from build123d import *

# Parameters (mm, degrees)
SKETCH1_R           = 1.35
BOSS_EXTRUDE1_DEPTH = 10
SKETCH2_R           = 25
BOSS_EXTRUDE2_DEPTH = 2
CIRPATTERN1_COUNT   = 2
CIRPATTERN1_ANGLE   = 134.8
CIRPATTERN2_COUNT   = 2
CIRPATTERN2_ANGLE   = 225.2
FILLET1_R           = 7


with BuildPart() as part:
    # Sketch1 → Boss-Extrude1 (new body)
    with BuildSketch(Plane.XY):
        with BuildLine():
            Line((3.15, 3.85), (3.15, -1.35))
            ThreePointArc((3.15, -1.35), (0, -4.5), (-3.15, -1.35))
            Line((-3.15, -1.35), (-3.15, 3.85))
            ThreePointArc((-3.15, 3.85), (0, 7), (3.15, 3.85))
        make_face()
        Circle(SKETCH1_R, mode=Mode.SUBTRACT)
    boss_extrude1 = extrude(amount=BOSS_EXTRUDE1_DEPTH)

    # Sketch2 → Boss-Extrude2 (add)
    with BuildSketch(Plane.XY.offset(10)):
        with Locations((0, 26.766568047)):
            Circle(SKETCH2_R)
    extrude(amount=-BOSS_EXTRUDE2_DEPTH)

    # CirPattern1: Boss-Extrude1 ×2 about axis
    cirpattern1_axis = Axis((0, 26.766568047, 0), (0, 0, 1))
    for i in range(1, CIRPATTERN1_COUNT):
        add(boss_extrude1.rotate(cirpattern1_axis, i * CIRPATTERN1_ANGLE / (CIRPATTERN1_COUNT - 1)))

    # CirPattern2: Boss-Extrude1 ×2 about axis
    cirpattern2_axis = Axis((0, 26.766568047, 0), (0, 0, 1))
    for i in range(1, CIRPATTERN2_COUNT):
        add(boss_extrude1.rotate(cirpattern2_axis, i * CIRPATTERN2_ANGLE / (CIRPATTERN2_COUNT - 1)))

    # Fillet1
    # the kernel refuses this fillet: 7 mm, written as the material it adds along each edge
    with BuildSketch(Plane(origin=(-19.817488489, 42.006881364, 8), x_dir=(-0.53269115848809, -0.8463097126162599, 0), z_dir=(0, 0, 1))) as fillet1_piece_1:
        with BuildLine():
            CenterArc((5.338447362, -6.96923168), FILLET1_R, 95.374025281, 58.803015478)
            Line((-0.962562709, -3.920088835), (-1.592663716, -3.61517455))
            ThreePointArc((-1.592663716, -3.61517455), (-1.407138142, -3.082948514), (-0.683108314, 0.152849703))
            Line((-0.683108314, 0.152849703), (0.06555988, 0.696923168))
            ThreePointArc((0.06555988, 0.696923168), (2.341424281, 0.590113144), (4.617288683, 0.696923168))
            Line((4.617288683, 0.696923168), (4.682848563, 0))
        make_face()
    extrude(amount=2)
    with BuildSketch(Plane(origin=(-15.378292966, 46.477177004, 8), x_dir=(0.8425702330097088, 0.5385864855767968, 0), z_dir=(0, 0, 1)), Plane(origin=(19.817488489, 42.006881364, 8), x_dir=(0.532691158488102, -0.8463097126162524, 0), z_dir=(0, 0, 1))) as fillet1_piece_2:
        with BuildLine():
            CenterArc((5.338447362, 6.96923168), FILLET1_R, 205.822959241, 58.803015478)
            Line((-0.962562709, 3.920088835), (-1.592663716, 3.61517455))
            ThreePointArc((-1.592663716, 3.61517455), (-1.407138142, 3.082948514), (-0.683108314, -0.152849703))
            Line((-0.683108314, -0.152849703), (0.06555988, -0.696923168))
            ThreePointArc((0.06555988, -0.696923168), (2.341424281, -0.590113144), (4.617288683, -0.696923168))
            Line((4.617288683, -0.696923168), (4.682848563, 0))
        make_face()
    extrude(amount=2)
    with BuildSketch(Plane(origin=(15.378292966, 46.477177004, 8), x_dir=(0.7239706283099918, 0.6898307976195582, 0), z_dir=(0, 0, 1)), Plane(origin=(3.15, 1.96581201, 8), x_dir=(-0.020650724563576823, -0.9997867510499423, 0), z_dir=(0, 0, 1))) as fillet1_piece_3:
        with BuildLine():
            CenterArc((5.495161337, 6.846342989), FILLET1_R, 199.169842212, 58.803015478)
            Line((-1.116684038, 4.547756306), (-1.777868575, 4.317897638))
            ThreePointArc((-1.777868575, 4.317897638), (-1.131431398, 2.133158264), (-0.692451691, -0.102521492))
            Line((-0.692451691, -0.102521492), (0.014455507, -0.699850726))
            ThreePointArc((0.014455507, -0.699850726), (3.329560424, -0.631376805), (3.890673543, -0.684634299))
            Line((3.890673543, -0.684634299), (4.03653607, 0))
        make_face()
    extrude(amount=2)
    with BuildSketch(Plane(origin=(-3.15, 1.96581201, 8), x_dir=(0.020650724563576386, -0.9997867510499423, 0), z_dir=(0, 0, 1))) as fillet1_piece_4:
        with BuildLine():
            CenterArc((5.495161337, -6.846342989), FILLET1_R, 102.02714231, 58.803015478)
            Line((-1.116684038, -4.547756306), (-1.777868575, -4.317897638))
            ThreePointArc((-1.777868575, -4.317897638), (-1.131431398, -2.133158264), (-0.692451691, 0.102521492))
            Line((-0.692451691, 0.102521492), (0.014455507, 0.699850726))
            ThreePointArc((0.014455507, 0.699850726), (3.329560424, 0.631376805), (3.890673543, 0.684634299))
            Line((3.890673543, 0.684634299), (4.03653607, 0))
        make_face()
    extrude(amount=2)


solid = part.part
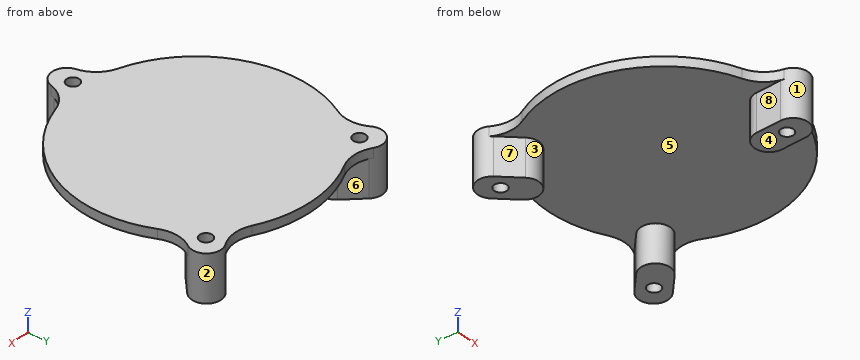
Work out the finished part from the listing and answer in its coordinate system (mm). Face numbers are marked on the shaded views. A direction names the side the tool comes from. Round coordinates to 2 decimals unless told otherwise and drop trailing zeros. Loops run counter-clockwise (first coordinate to the right, second up) from the corner with the lowest first, then second, coordinate; pieces in that order, holes last. Notation, with made-up numbers: (67, -18.75) -> (110, -18.75) arc R19 ccw to (110, -14.75) -> close; hole circle Ø6 at (-24, 47). An arc over 180 degrees is marked (long way). Use one line per item in the form item = value.
(1) Find section C-C on y = 0. Give the vertices of the cut face in (x, z).
Answer list:
outline = (-3.92, 8) -> (-3.15, 8) -> (-3.15, 0) -> (-1.35, 0) -> (-1.35, 10) -> (-3.92, 10) -> close; (1.35, 0) -> (3.15, 0) -> (3.15, 8) -> (3.92, 8) -> (3.92, 10) -> (1.35, 10) -> close
(2) Straight lines are drawn through the part: line 1 (Y direction, x = 0, z = 3.25); line 2 (Z direction, x = -9, y = 19); line 3 (X direction, y = 0, z = 7). For each, find the intervals that lie inside material, in ascending order.
Answer list:
line_1 = -4.5 to -1.35, 1.35 to 7
line_2 = 8 to 10
line_3 = -3.15 to -1.35, 1.35 to 3.15
(3) Find section B-B on z = 7.25. Give the vertices of the cut face in (x, y).
Answer list:
outline = (-22.17, 44.34) -> (-18.48, 40.68) arc R3.15 ccw to (-14.04, 45.15) -> (-17.73, 48.81) arc R3.15 ccw to start; (-3.15, -1.35) arc R3.15 ccw to (3.15, -1.35) -> (3.15, 3.85) arc R3.15 ccw to (-3.15, 3.85) -> close; (14.04, 45.15) arc R3.15 ccw to (18.48, 40.68) -> (22.17, 44.34) arc R3.15 ccw to (17.73, 48.81) -> close; hole circle Ø2.7 at (-18.99, 45.63); hole circle Ø2.7 at (0, 0); hole circle Ø2.7 at (18.99, 45.63)
(4) Find section A-A on x = 0. Give the vertices of the cut face in (y, z).
Answer list:
outline = (-4.5, 0) -> (-1.35, 0) -> (-1.35, 10) -> (-4.5, 10) -> close; (1.35, 0) -> (7, 0) -> (7, 8) -> (51.77, 8) -> (51.77, 10) -> (1.35, 10) -> close
(5) A tool of negligible diameter and unlimited length cuts with its end or side. For the marked faces 5, 6, 7 and 8, from which of +Z, -Z, +X, -X, +Y, -Y can it reach the whole face along a straight path? Write none if from no direction.
Answer list:
face_5 = -Z
face_6 = -Z, +Y
face_7 = -Z, -X, -Y
face_8 = -Z, -X, +Y, -Y
(6) Find section D-D on x = -16. Give the vertices of the cut face in (y, z), then the cut area to 3 significant figures.
Answer list:
outline = (7.56, 8) -> (39.78, 8) -> (39.78, 0) -> (47.09, 0) -> (47.09, 8) -> (48.36, 8) -> (48.36, 10) -> (7.56, 10) -> close
area = 140 mm2
(7) Flat-ended cylindrical pins translate along their axes: P1, Ø6, axis at x = 19.5, z = 8, coming from the +Y side; P2, Ø6, axis at x = -9.5, y = 34.5, coming from the -Z side; P3, Ø5.5, axis at y = 2.5, z = 5, coming from the +X side. Find the tip coordinate at first contact, or state that the pin passes through.
Answer list:
P1 = 49.73
P2 = 8
P3 = 3.15
(8) For a pull along X with two mould halves and no side action, classify the marked faces 1, 2, 3 and 4 as released by +X, released by -X, zero draft, split by the parting line, or undercut.
Answer list:
face_1 = split by the parting line
face_2 = undercut
face_3 = undercut
face_4 = zero draft
